Job drawing, mm, ordinate dimensions from the low corner. One solid piece. A direction names the side the tool comes from. Round coordinates to 2 decimals unless told otherwise and drop trailing zeros. Order: outer loops, then holes, each group sorted by start corner. A loop starts at its lowest first (then second) coordinate and runs counter-clockwise, first axis right, second up. Notation, with made-up numbers: (57, 29.25) -> (81, 29.25) arc R18 ccw to (81, 53.25) -> close; hole circle Ø2 at (3, 35). An arc over 180 degrees is marked (long way). Use CSV: the item, a comma, the result in double quotes.
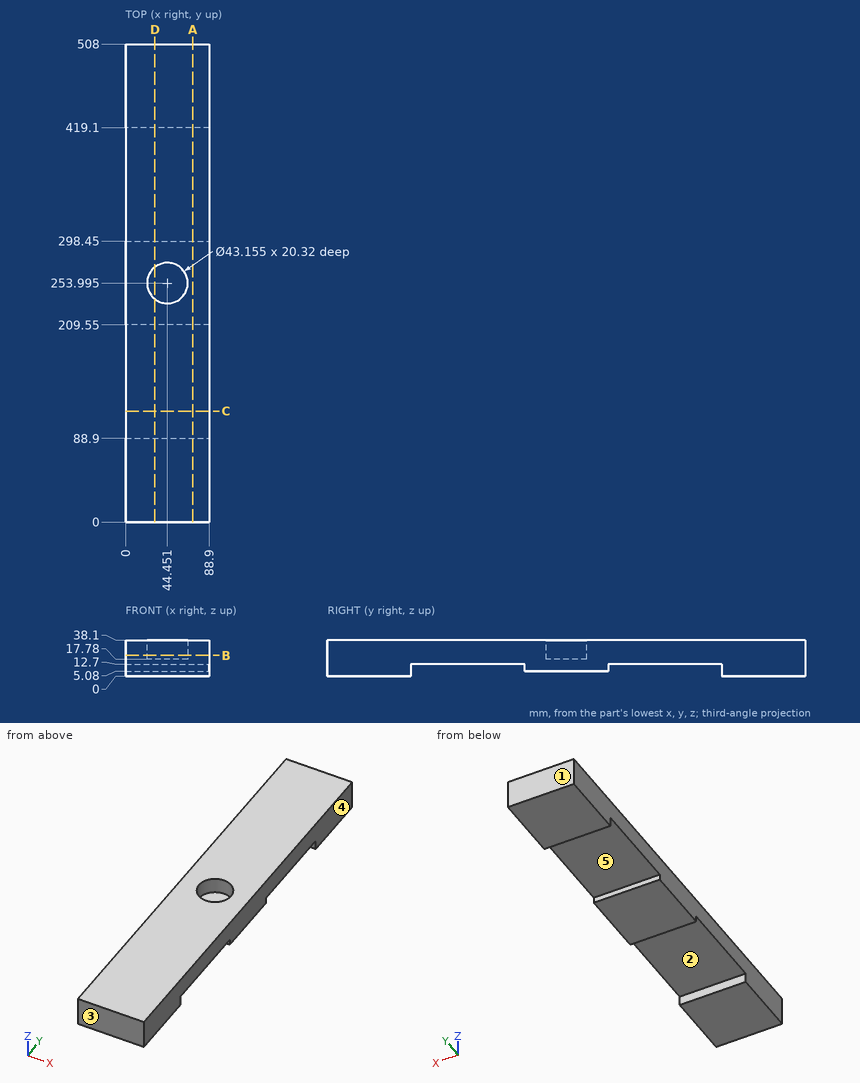
(1) Cut at A-A, the plane x = 71.5. Give the cut face in (y, z), then the cut area to 3 significant figures.
Reply:
outline,"(0, 0) -> (88.9, 0) -> (88.9, 12.7) -> (209.55, 12.7) -> (209.55, 5.08) -> (298.45, 5.08) -> (298.45, 12.7) -> (419.1, 12.7) -> (419.1, 0) -> (508, 0) -> (508, 38.1) -> (0, 38.1) -> close"
area,"15,800 mm2"
(2) Pull direction Y, two halves, no side cores. Call the marked faces 1, 2 and 3: released by +Y, released by -Y, zero draft, split by the parting line, or undercut.
Reply:
face 1,"released by +Y"
face 2,"undercut"
face 3,"released by -Y"
(3) Which spindle directions (+Z, -Z, +X, -X, +Y, -Y) get a long thin tool onto all of the face, cutting with end or side? Do the marked faces 4 and 5. Say none if no direction does.
Reply:
face 4,"+Z, -Z, +X, +Y, -Y"
face 5,"-Z, +X, -X"
(4) Drop flat-ended pins along their axis: P1, Ø1.5, axis at y = 364.5, z = 21.5, coming from the -X side; P2, Ø10, axis at x = 75, y = 114.5, coming from the -Z side; P3, Ø13, axis at x = 50.5, y = 260, coming from the +Z side. Give the stop position or say it passes through.
Reply:
P1,"x = 0"
P2,"z = 12.7"
P3,"z = 17.78"
(5) Cut at D-D, the plane x = 31. Give the cut face in (y, z).
Reply:
outline,"(0, 0) -> (88.9, 0) -> (88.9, 12.7) -> (209.55, 12.7) -> (209.55, 5.08) -> (298.45, 5.08) -> (298.45, 12.7) -> (419.1, 12.7) -> (419.1, 0) -> (508, 0) -> (508, 38.1) -> (270.87, 38.1) -> (270.87, 17.78) -> (237.12, 17.78) -> (237.12, 38.1) -> (0, 38.1) -> close"
(6) Probe probe 1 along Z at (x, y) = (13.5, 368); probe 2 along Z at (x, y) = (85, 282); probe 3 along X at (y, z) = (234, 21) (1 decimal). List the from-to ranges inside material, lowest first. Write a range as [from, to].
Reply:
probe 1,"[12.7, 38.1]"
probe 2,"[5.08, 38.1]"
probe 3,"[0, 36.3], [52.6, 88.9]"
(7) Cut at C-C, the plane y = 118. Give the cut face in (x, z), then the cut area to 3 significant figures.
Reply:
outline,"(0, 12.7) -> (88.9, 12.7) -> (88.9, 38.1) -> (0, 38.1) -> close"
area,"2,260 mm2"
(8) Cut at B-B, the plane z = 22. Give the cut face in (x, y) (1 decimal), then the cut area to 3 significant figures.
Reply:
outline,"(0, 0) -> (88.9, 0) -> (88.9, 508) -> (0, 508) -> close; hole circle Ø43.2 at (44.5, 254)"
area,"43,700 mm2"
